Geometry check sheet. Reference: the model listing, model coordinates, mm. A direction names the side the tool comes from. Round coordinates to 2 decimals unless told otherwise and drop trailing zeros. Write each loop counter-clockwise with the first axis right and the second up, starting at its lowest first coordinate (ties: lowest second). Pieces come first, ordered by that corner, then holes.
Item 1: Access from +Z, -Z, +X, -X, +Y, -Y to the whole of each face (thin tool, end or side, straight path). Record for faces 1 (the face through (7.9, 0.5, -7.481)), 2 (the face through (-2, 0, 1)).
Item 2: Draft check along X on faces 3 (the face through (-21, -3, -11.882)), 4 (the face through (-8.5, 0.5, -15.682)). Enter one of: pulls with the +X half, pulls with the -X half, needs draft (parallel to the pull), parting line crosses it, or undercut.
Item 3: Cross-section at B-B (z = 10). Enter the section's corners in (x, y).
Item 4: Cross-section at D-D (x = 2.5). Enter the section's corners in (y, z), then the cut area to 3 significant figures.
Item 5: Scan lines: probe 1 along X at (y, z) = (0.55, -17); probe 2 along X at (y, z) = (0.5, -12); probe 3 along X at (y, z) = (-4.2, 16). Record each from-to range of solid material in increasing order.
Item 6: Depth check by flat-ended pin: P1, Ø7.5, axis at x = -15, z = 17, coming from the -Y side; P2, Ø12, axis at x = 13.5, z = -13, coming from the -Y side; P3, Ø3, axis at x = 14.5, z = -1, coming from the -Y side; P4, Ø1, axis at y = -1, z = -1, coming from the -X side. Enter the tip coordinate at first touch or a pass-through.
Item 7: Cross-section at A-A (x = -9.5). Enter the section's corners in (y, z).
Item 8: Cross-section at C-C (y = -3.55). Enter the section's corners in (x, z), then the cut area to 3 significant figures.
from build123d import *

# Parameters (mm, degrees)
SKETCH_1_W          = 43.6316
SKETCH_1_H          = 45
SKETCH_1_RX         = 1.5
SKETCH_1_RY         = 1.5
SKETCH_1_W_2        = 5.2
SKETCH_1_H_2        = 5.2
EXTRUDE_1_DEPTH     = 1
SKETCH_3_R          = 4
SKETCH_3_R_2        = 1.5
EXTRUDE_3_DEPTH     = 1.2
SKETCH_4_W          = 43.6316
SKETCH_4_H          = 45
SKETCH_4_W_2        = 39.6316
SKETCH_4_H_2        = 41
EXTRUDE_4_DEPTH     = 5
SKETCH_5_W          = 2
SKETCH_5_H          = 25
CUT_EXTRUDE_1_DEPTH = 5


with BuildPart() as part:
    # Эскиз1 → Бобышка-Вытянуть1 (new body)
    with BuildSketch(Plane(origin=(0, 0, 0), x_dir=(1, 0, 0), z_dir=(0, 1, 0))):
        with Locations((-0.355064662, -0.618327068)):
            Rectangle(SKETCH_1_W, SKETCH_1_H)
        with Locations(Location((-17.170864662, 16.881672932), (0, 0, 90))):
            Ellipse(SKETCH_1_RX, SKETCH_1_RY, mode=Mode.SUBTRACT)
        with Locations(Location((-17.170864662, -18.118327068), (0, 0, 90))):
            Ellipse(SKETCH_1_RX, SKETCH_1_RY, mode=Mode.SUBTRACT)
        with Locations(Location((16.629135338, 16.881672932), (0, 0, 90))):
            Ellipse(SKETCH_1_RX, SKETCH_1_RY, mode=Mode.SUBTRACT)
        with Locations(Location((16.629135338, -18.118327068), (0, 0, 90))):
            Ellipse(SKETCH_1_RX, SKETCH_1_RY, mode=Mode.SUBTRACT)
        with Locations((-8.470864662, 13.081672932)):
            Rectangle(SKETCH_1_W_2, SKETCH_1_H_2, mode=Mode.SUBTRACT)
        with Locations((-8.470864662, 6.981672932)):
            Rectangle(SKETCH_1_W_2, SKETCH_1_H_2, mode=Mode.SUBTRACT)
        with Locations((-8.470864662, 0.881672932)):
            Rectangle(SKETCH_1_W_2, SKETCH_1_H_2, mode=Mode.SUBTRACT)
        with Locations((-8.470864662, -5.218327068)):
            Rectangle(SKETCH_1_W_2, SKETCH_1_H_2, mode=Mode.SUBTRACT)
        with Locations((-8.470864662, -11.318627068)):
            Rectangle(SKETCH_1_W_2, SKETCH_1_H_2, mode=Mode.SUBTRACT)
        with Locations((7.929135338, 10.081372932)):
            Rectangle(SKETCH_1_W_2, SKETCH_1_H_2, mode=Mode.SUBTRACT)
        with Locations((7.929135338, 3.981372932)):
            Rectangle(SKETCH_1_W_2, SKETCH_1_H_2, mode=Mode.SUBTRACT)
        with Locations((7.929135338, -2.118627068)):
            Rectangle(SKETCH_1_W_2, SKETCH_1_H_2, mode=Mode.SUBTRACT)
        with Locations((7.929135338, -8.218627068)):
            Rectangle(SKETCH_1_W_2, SKETCH_1_H_2, mode=Mode.SUBTRACT)
        with Locations((7.929135338, -14.318627068)):
            Rectangle(SKETCH_1_W_2, SKETCH_1_H_2, mode=Mode.SUBTRACT)
    extrude(amount=EXTRUDE_1_DEPTH)

    # Эскиз3 → Бобышка-Вытянуть3 (add)
    with BuildSketch(Plane.XZ):
        with Locations((-17.170864662, 18.118327068)):
            Circle(SKETCH_3_R)
        with Locations((-17.170864662, 18.118327068)):
            Circle(SKETCH_3_R_2, mode=Mode.SUBTRACT)
        with Locations((16.629135338, 18.118327068)):
            Circle(SKETCH_3_R)
        with Locations((16.629135338, 18.118327068)):
            Circle(SKETCH_3_R_2, mode=Mode.SUBTRACT)
        with Locations((-17.170864662, -16.881672932)):
            Circle(SKETCH_3_R)
        with Locations((-17.170864662, -16.881672932)):
            Circle(SKETCH_3_R_2, mode=Mode.SUBTRACT)
        with Locations((16.629135338, -16.881672932)):
            Circle(SKETCH_3_R)
        with Locations((16.629135338, -16.881672932)):
            Circle(SKETCH_3_R_2, mode=Mode.SUBTRACT)
    extrude(amount=EXTRUDE_3_DEPTH)

    # Эскиз4 → Бобышка-Вытянуть4 (add)
    with BuildSketch(Plane.XZ):
        with Locations((-0.355064662, 0.618327068)):
            Rectangle(SKETCH_4_W, SKETCH_4_H)
        with Locations((-0.355064662, 0.618327068)):
            Rectangle(SKETCH_4_W_2, SKETCH_4_H_2, mode=Mode.SUBTRACT)
    extrude(amount=EXTRUDE_4_DEPTH)

    # Эскиз5 → Вырез-Вытянуть1 (cut)
    with BuildSketch(Plane.XZ.offset(5)):
        with Locations((-21.170864662, 0.618327068)):
            Rectangle(SKETCH_5_W, SKETCH_5_H)
    extrude(amount=-CUT_EXTRUDE_1_DEPTH, mode=Mode.SUBTRACT)


solid = part.part
Resolved:
1. face 1: +Y, -Y
1. face 2: -Y
2. face 3: needs draft
2. face 4: undercut
3. outline: (-22.17, 0) - (-11.07, 0) - (-11.07, 1) - (-22.17, 1) - close; (-5.87, 0) - (5.33, 0) - (5.33, 1) - (-5.87, 1) - close; (10.53, 0) - (19.46, 0) - (19.46, -5) - (21.46, -5) - (21.46, 1) - (10.53, 1) - close
4. outline: (-5, -21.88) - (1, -21.88) - (1, 23.12) - (-5, 23.12) - (-5, 21.12) - (0, 21.12) - (0, -19.88) - (-5, -19.88) - close
4. area: 65.0 mm2
5. probe 1: x = -22.17 to -18.67, -15.68 to 15.13, 18.12 to 21.46
5. probe 2: x = -22.17 to -11.07, -5.87 to 5.33, 10.53 to 21.46
5. probe 3: x = -22.17 to -20.17, 19.46 to 21.46
6. P1: stops at y = -1.2
6. P2: stops at y = -5
6. P3: stops at y = 0
6. P4: stops at x = 19.46
7. outline: (-5, -21.88) - (1, -21.88) - (1, -15.68) - (0, -15.68) - (0, -19.88) - (-5, -19.88) - close; (-5, 21.12) - (0, 21.12) - (0, 13.92) - (1, 13.92) - (1, 23.12) - (-5, 23.12) - close; (0, -10.48) - (1, -10.48) - (1, -9.58) - (0, -9.58) - close; (0, -4.38) - (1, -4.38) - (1, -3.48) - (0, -3.48) - close; (0, 1.72) - (1, 1.72) - (1, 2.62) - (0, 2.62) - close; (0, 7.82) - (1, 7.82) - (1, 8.72) - (0, 8.72) - close
8. outline: (-22.17, -21.88) - (21.46, -21.88) - (21.46, 23.12) - (-22.17, 23.12) - (-22.17, 13.12) - (-20.17, 13.12) - (-20.17, 21.12) - (19.46, 21.12) - (19.46, -19.88) - (-20.17, -19.88) - (-20.17, -11.88) - (-22.17, -11.88) - close
8. area: 289 mm2
